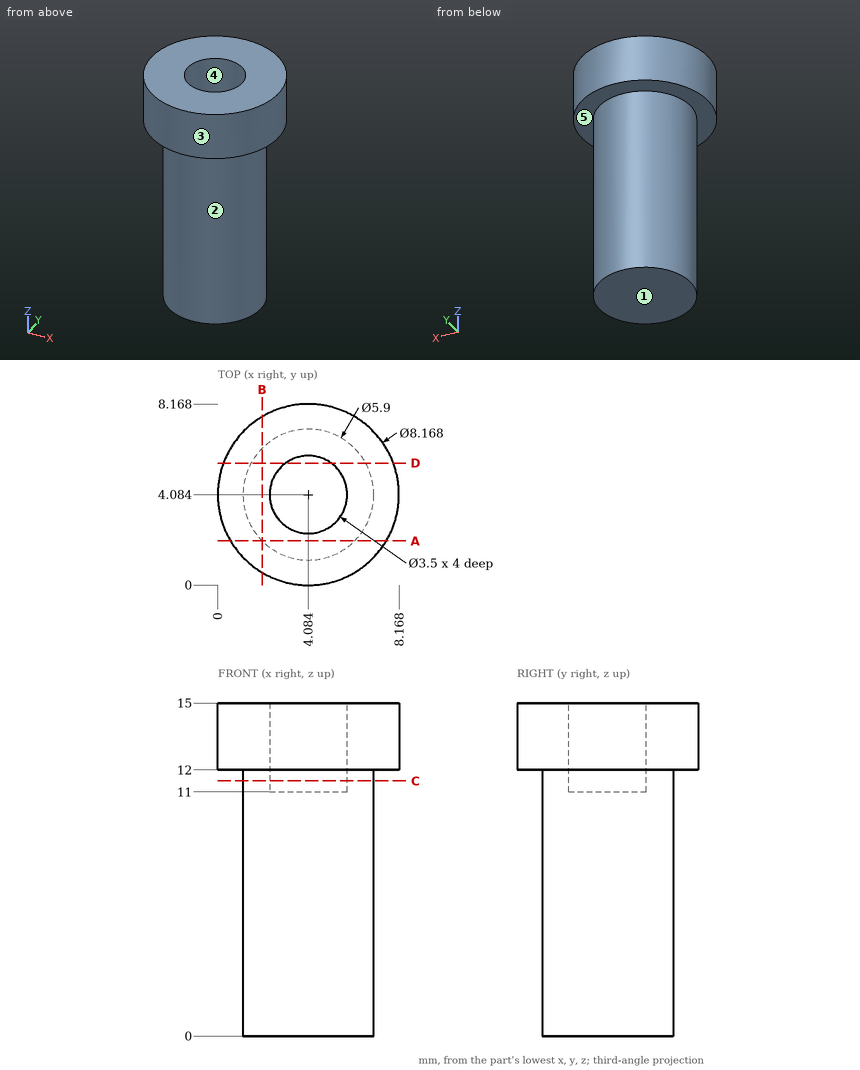
Source: three-view drawing plus pictorial views. Frame: mm from the lowest corner of the part. A direction names the side the tool comes from. Give positions to 0.01 mm unless a question says otherwise; leave off trailing zeros. Order: outer loops, then holes, each group sorted by start corner. A loop starts at its lowest first (then second) coordinate and runs counter-clockwise, first axis right, second up. Notation, with made-up numbers: M 81,-15.5 L 127,-15.5 A16 cw 127,-10.5 Z; hole C 85,-11 d7. An arc over 180 degrees is marked long. Return JSON: item names as keys, results as strings.
Item 1: Access query for the marked faces 1 and 2. Directions: +Z, -Z, +X, -X, +Y, -Y. A direction counts if a zero-diameter tool reaches every point of the face in a straight line with its end or side. Return the directions, or none.
Solutions:
{"face 1": "-Z, +X, -X, +Y, -Y", "face 2": "-Z"}
Item 2: Cut plane A-A (y = 2). Return loops of the section in (x, z).
Solutions:
{"outline": "M 0.57,12 L 2,12 L 2,0 L 6.17,0 L 6.17,12 L 7.6,12 L 7.6,15 L 0.57,15 Z"}
Item 3: Ray query, probe 1 along Y at (x, z) = (4, 14.75); probe 2 along Z at (x, y) = (7, 5); probe 3 along Z at (x, y) = (3, 3.75). Return the intervals inside material, ascending.
Solutions:
{"probe 1": "0 to 2.34, 5.83 to 8.17", "probe 2": "12 to 15", "probe 3": "0 to 11"}
Item 4: Cut plane D-D (y = 5.5). Return loops of the section in (x, z).
Solutions:
{"outline": "M 0.25,12 L 1.5,12 L 1.5,0 L 6.67,0 L 6.67,12 L 7.91,12 L 7.91,15 L 5.11,15 L 5.11,11 L 3.06,11 L 3.06,15 L 0.25,15 Z"}
Item 5: Cut plane C-C (z = 11.5). Return loops of the section in (x, y).
Solutions:
{"outline": "C 4.08,4.08 d5.9; hole C 4.08,4.08 d3.5"}
Item 6: First-contact query: P1, Ø1.5, axis at x = 3, z = 2, coming from the +Y side; P2, Ø4, axis at y = 3.5, z = 4.5, coming from the -X side. Flat tips, straight axial feed; report the tip coordinate or a pass-through.
Solutions:
{"P1": "y = 7.02", "P2": "x = 1.13"}
Item 7: Pull-direction query (Y, two-part tool) for the marked faces 3, 4 and 5; classes: +Y half, -Y half, draft (parallel to the pull), parting line (faces both ways), or undercut.
Solutions:
{"face 3": "parting line", "face 4": "undercut", "face 5": "draft"}
